Could you check a few things on this model? Use its own coordinates, in mm. A direction names the side the tool comes from. Coordinates: 2 decimals unless noted, no trailing zeros. Loops run counter-clockwise (first coordinate to the right, second up) from the corner with the lowest first, then second, coordinate; pieces in that order, holes last.
1) Imagine slicing it at A-A on x = -15.5. Please give me the cut outline in (y, z).
2) Will these pins go through, and if not, where does the flat tip stop? P1, Ø5, axis at x = -12, y = 40.5, coming from the +Z side; P2, Ø3, axis at x = 15.5, z = -5.5, coming from the +Y side.
3) For faces 4 (the face through (-28, 13, 10)), 5 (the face through (11.15, 53, 12)), 6 (the face through (-31.458, 33.247, -1.689)), 7 (the face through (17.235, 53.028, -5.728)), 8 (the face through (0, 3, 2)), which set-ups out of +Z, -Z, +X, -X, +Y, -Y let a thin tool reach every point of the face, with its end or its side?
4) If I drill on line 1 along X through (y, z) = (53.1, -5.5); line 2 along Y through (x, z) = (13, -9.5); line 3 along X through (y, z) = (17.5, 9.5), over which ranges is the centre line in solid material (lowest first)?
5) Imagine slicing it at C-C on x = 0. Please give me the cut outline in (y, z).
6) Thinking about a two-plate mould opening in Y: for faces 1 (the face through (0, 0, 0)), 2 (the face through (-0.245, 52.986, -1.147)), 3 (the face through (0, 51, -5)), which applies, released by +Y, released by -Y, zero draft, split by the parting line, or undercut?
7) Imagine slicing it at D-D on y = 41. Please give me the cut outline in (x, z).
8) Imagine slicing it at B-B on z = -10. Please give me the cut outline in (x, y).
```python
from build123d import *

# Parameters (mm, degrees)
CROQUIS1_W              = 70
CROQUIS1_H              = 30
SALIENTE_EXTRUIR1_DEPTH = 55
CROQUIS5_W              = 44
CROQUIS5_H              = 48
CORTAR_EXTRUIR3_DEPTH   = 27
CORTAR_EXTRUIR4_REACH   = 65.647
CROQUIS6_R              = 11.15
CORTAR_EXTRUIR5_START   = -4
CROQUIS7_W              = 22.3
CROQUIS7_H              = 5
CORTAR_EXTRUIR5_DEPTH   = 4
CROQUIS9_R              = 4.15
CORTAR_EXTRUIR6_DEPTH   = 27
REDONDEO1_R             = 1
CORTAR_EXTRUIR7_DEPTH   = 1
CORTAR_EXTRUIR8_REACH   = 68.895
CROQUIS11_R             = 1.75
CORTAR_EXTRUIR9_REACH   = 82.616


with BuildPart() as part:
    # Croquis1 → Saliente-Extruir1 (new body)
    with BuildSketch(Plane(origin=(0, 0, 0), x_dir=(1, 0, 0), z_dir=(0, 1, 0))):
        Rectangle(CROQUIS1_W, CROQUIS1_H)
    extrude(amount=SALIENTE_EXTRUIR1_DEPTH)

    # Croquis5 → Cortar-Extruir3 (cut)
    with BuildSketch(Plane.XY.offset(15)):
        with Locations((0, 27)):
            Rectangle(CROQUIS5_W, CROQUIS5_H)
    extrude(amount=-CORTAR_EXTRUIR3_DEPTH, mode=Mode.SUBTRACT)

    # Croquis6 → Cortar-Extruir4 (cut, up to next)
    with BuildSketch(Plane.XZ.offset(-51), mode=Mode.PRIVATE) as cortar_extruir4_sk1:
        with Locations((0, 10)):
            Circle(CROQUIS6_R)
    cortar_extruir4_tool1 = extrude(cortar_extruir4_sk1.sketch, amount=-CORTAR_EXTRUIR4_REACH, mode=Mode.PRIVATE) & part.part
    add(cortar_extruir4_tool1.solids().sort_by_distance((0, 51, 10))[0], mode=Mode.SUBTRACT)

    # Croquis7 → Cortar-Extruir5 (cut)
    with BuildSketch(Plane(origin=(0, 55, 0), x_dir=(1, 0, 0), z_dir=(0, 1, 0)).offset(CORTAR_EXTRUIR5_START)):
        with Locations((0, -12.5)):
            Rectangle(CROQUIS7_W, CROQUIS7_H)
    extrude(amount=CORTAR_EXTRUIR5_DEPTH, mode=Mode.SUBTRACT)

    # Croquis9 → Cortar-Extruir6 (cut)
    with BuildSketch(Plane(origin=(0, 0, -15), x_dir=(-1, 0, 0), z_dir=(0, 0, -1))):
        with Locations((-27.5, 32)):
            Circle(CROQUIS9_R)
        with Locations((27.5, 32)):
            Circle(CROQUIS9_R)
    extrude(amount=-CORTAR_EXTRUIR6_DEPTH, mode=Mode.SUBTRACT)

    # Redondeo1
    redondeo1_edges = [part.edges().sort_by_distance(p)[0] for p in [
        (-35, 55, 0),
        (-23.075, 55, 15),
        (-22, 27, 15),
        (0, 3, 15),
        (22, 27, 15),
        (16.575, 51, 15),
        (0, 55, -1.15),
        (23.075, 55, 15),
        (11.15, 51, 12.5),
        (35, 55, 0),
        (11.15, 55, 12.5),
        (11.15, 53, 15),
        (0, 51, -1.15),
        (-16.575, 51, 15),
        (-11.15, 51, 12.5),
        (-11.15, 55, 12.5),
        (-11.15, 53, 15),
        (0, 55, -15),
        (35, 27.5, 15),
        (-35, 27.5, 15),
        (-35, 27.5, -15),
        (35, 27.5, -15),
    ]]
    fillet(redondeo1_edges, radius=REDONDEO1_R)

    # Croquis10 → Cortar-Extruir7 (cut)
    with BuildSketch(Plane.XY.offset(15)):
        with BuildLine():
            Line((30.192307692, 11.128219757), (30.192307692, 10.512835142))
            Line((30.192307692, 10.512835142), (28.151442308, 10.512835142))
            Line((28.151442308, 10.512835142), (27.828125, 8.934710142))
            add(Edge.make_bspline(
                [(27.828125, 8.934710142), (27.891649356, 8.952247751), (28.014717749, 8.986224094), (28.196363225, 9.023948272), (28.368807002, 9.046689033), (28.480707637, 9.049794137), (28.534855769, 9.05129668)],
                knots=[0, 0, 0, 0, 1.100273476, 2.13160584, 3.095893838, 4, 4, 4, 4], degree=3))
            add(Edge.make_bspline(
                [(28.534855769, 9.05129668), (28.601856466, 9.049846505), (28.733596576, 9.046995098), (28.926349056, 9.019614784), (29.110348302, 8.976517788), (29.285209508, 8.916311179), (29.451256166, 8.839323065), (29.606960557, 8.743151739), (29.754659836, 8.630808885), (29.891704283, 8.501646008), (30.016031669, 8.359494665), (30.125344794, 8.2066526), (30.218194949, 8.044605179), (30.292870528, 7.871804136), (30.352500816, 7.690159873), (30.39218995, 7.49776116), (30.418618594, 7.296421525), (30.421571256, 7.158756548), (30.423076923, 7.088556296)],
                knots=[0, 0, 0, 0, 1.052922333, 2.070308379, 3.05430497, 4.020497103, 4.973039431, 5.925935799, 6.892292201, 7.88610001, 8.88166317, 9.857072816, 10.836096531, 11.812156883, 12.81219415, 13.836441305, 14.89672472, 16, 16, 16, 16], degree=3))
            add(Edge.make_bspline(
                [(30.423076923, 7.088556296), (30.421936794, 7.039661061), (30.419671944, 6.942531368), (30.408154365, 6.798284167), (30.385978852, 6.657090739), (30.35620561, 6.518932353), (30.317561465, 6.384070572), (30.27078023, 6.252119381), (30.213529897, 6.123900055), (30.150733254, 5.998199378), (30.080025006, 5.87785908), (30.001547565, 5.76531796), (29.918635294, 5.658887763), (29.82942149, 5.559709935), (29.733076927, 5.46843619), (29.630768413, 5.384524851), (29.523312323, 5.306556856), (29.409046193, 5.237697093), (29.290516222, 5.174332025), (29.166010707, 5.122348818), (29.038363792, 5.075873627), (28.905738291, 5.038828723), (28.768434612, 5.009801486), (28.626226426, 4.990086171), (28.479859563, 4.975726564), (28.380645256, 4.974827666), (28.330528846, 4.974373604)],
                knots=[0, 0, 0, 0, 1.056347294, 2.098418968, 3.122841568, 4.141288669, 5.149314143, 6.15115421, 7.162517403, 8.180376062, 9.185164535, 10.17417709, 11.141909838, 12.097768115, 13.052685741, 14.0056014, 14.954263652, 15.917497458, 16.885230207, 17.854509472, 18.828990115, 19.81800267, 20.826176721, 21.857883937, 22.917946725, 24, 24, 24, 24], degree=3))
            add(Edge.make_bspline(
                [(28.330528846, 4.974373604), (28.270744536, 4.975557897), (28.153125969, 4.977887855), (27.980804997, 5.002262401), (27.81500853, 5.037171972), (27.657071214, 5.089691292), (27.505577619, 5.155498083), (27.362567246, 5.238668663), (27.224385916, 5.332918555), (27.096650995, 5.444142017), (26.978097658, 5.565711758), (26.871972214, 5.697639142), (26.777457511, 5.837746757), (26.696067088, 5.986715022), (26.626641908, 6.144152503), (26.572101929, 6.310649076), (26.528081891, 6.485334797), (26.509458885, 6.605597958), (26.5, 6.666681296)],
                knots=[0, 0, 0, 0, 1.0467383, 2.05933395, 3.04377827, 4.011590433, 4.970194871, 5.932262533, 6.905835911, 7.896367577, 8.894135286, 9.877477877, 10.858688626, 11.851381753, 12.8477658, 13.868841284, 14.917554742, 16, 16, 16, 16], degree=3))
            Line((26.5, 6.666681296), (27.038461538, 6.666681296))
            add(Edge.make_bspline(
                [(27.038461538, 6.666681296), (27.051710494, 6.60946452), (27.077175722, 6.4994907), (27.133071291, 6.34497983), (27.201412792, 6.207289732), (27.28267739, 6.084599018), (27.379620299, 5.977612165), (27.490242177, 5.88226863), (27.614266845, 5.796254123), (27.75208381, 5.724557951), (27.897477661, 5.663411516), (28.049650021, 5.622694325), (28.204457472, 5.594064223), (28.309163249, 5.591198347), (28.361778846, 5.589758219)],
                knots=[0, 0, 0, 0, 1.136247022, 2.183929868, 3.172523383, 4.106158343, 5.02341133, 5.958108904, 6.928429099, 7.938127109, 8.96079061, 9.975095812, 10.982467395, 12, 12, 12, 12], degree=3))
            add(Edge.make_bspline(
                [(28.361778846, 5.589758219), (28.413136179, 5.591165267), (28.514259189, 5.593935755), (28.663078709, 5.615259776), (28.806757922, 5.648101327), (28.943879105, 5.69724965), (29.076841744, 5.756983453), (29.202282493, 5.833637869), (29.323830283, 5.921855043), (29.437707083, 6.022923552), (29.542003282, 6.134300171), (29.634156632, 6.253404274), (29.710917055, 6.380461725), (29.775604099, 6.513272844), (29.82472404, 6.653293228), (29.859765722, 6.799866671), (29.880342394, 6.953355209), (29.883172989, 7.058045454), (29.884615385, 7.111392834)],
                knots=[0, 0, 0, 0, 1.027316725, 2.022795036, 3.002884548, 3.971462791, 4.93288096, 5.914575861, 6.907176829, 7.935150275, 8.956128384, 9.956726525, 10.942570165, 11.921478529, 12.907843606, 13.90538589, 14.932640048, 16, 16, 16, 16], degree=3))
            add(Edge.make_bspline(
                [(29.884615385, 7.111392834), (29.883486563, 7.159522694), (29.881277054, 7.253730047), (29.863224648, 7.391557258), (29.831824124, 7.521968188), (29.78824033, 7.645592589), (29.732904031, 7.762547061), (29.665281781, 7.872952307), (29.584104528, 7.975353164), (29.491375576, 8.069797542), (29.389790363, 8.156960185), (29.27760109, 8.231264333), (29.157155501, 8.293773906), (29.029904759, 8.347719046), (28.892822076, 8.386463181), (28.748622134, 8.415550985), (28.595747778, 8.432377321), (28.491226598, 8.434711986), (28.4375, 8.435912065)],
                knots=[0, 0, 0, 0, 1.045622112, 2.046656509, 3.013763289, 3.955457236, 4.890082067, 5.820317437, 6.762574623, 7.722996705, 8.69280354, 9.665887285, 10.63943826, 11.638615906, 12.663482002, 13.728887084, 14.832589034, 16, 16, 16, 16], degree=3))
            add(Edge.make_bspline(
                [(28.4375, 8.435912065), (28.390993265, 8.434916766), (28.294968656, 8.432861726), (28.147672381, 8.417730588), (27.992886571, 8.393320369), (27.831204578, 8.359743945), (27.66214085, 8.315804956), (27.486052163, 8.263151527), (27.302568277, 8.200199529), (27.178937893, 8.152658591), (27.115384615, 8.128219757)],
                knots=[0, 0, 0, 0, 0.817624296, 1.688186739, 2.600797293, 3.572016777, 4.590301741, 5.671205678, 6.80286297, 8, 8, 8, 8], degree=3))
            Line((27.115384615, 8.128219757), (27.730769231, 11.128219757))
            Line((27.730769231, 11.128219757), (30.192307692, 11.128219757))
        make_face()
    extrude(amount=-CORTAR_EXTRUIR7_DEPTH, mode=Mode.SUBTRACT)

    # Croquis11 → Cortar-Extruir8 (cut, up to next)
    with BuildSketch(Plane(origin=(0, 55, 0), x_dir=(1, 0, 0), z_dir=(0, 1, 0)), mode=Mode.PRIVATE) as cortar_extruir8_sk1:
        with Locations(Location((-15.5, 5.5, 0), (0, 0, 270))):
            Circle(CROQUIS11_R)
    cortar_extruir8_tool1 = extrude(cortar_extruir8_sk1.sketch, amount=-CORTAR_EXTRUIR8_REACH, mode=Mode.PRIVATE) & part.part
    # Croquis11 → Cortar-Extruir8 (cut, up to next)
    with BuildSketch(Plane(origin=(0, 55, 0), x_dir=(1, 0, 0), z_dir=(0, 1, 0)), mode=Mode.PRIVATE) as cortar_extruir8_sk2:
        with Locations(Location((15.5, 5.5, 0), (0, 0, 270))):
            Circle(CROQUIS11_R)
    cortar_extruir8_tool2 = extrude(cortar_extruir8_sk2.sketch, amount=-CORTAR_EXTRUIR8_REACH, mode=Mode.PRIVATE) & part.part
    add(cortar_extruir8_tool1.solids().sort_by_distance((-15.5, 55, -5.5))[0], mode=Mode.SUBTRACT)
    add(cortar_extruir8_tool2.solids().sort_by_distance((15.5, 55, -5.5))[0], mode=Mode.SUBTRACT)

    # Croquis14 → Cortar-Extruir9 (cut, up to next)
    with BuildSketch(Plane(origin=(-22, 0, 0), x_dir=(0, 0, -1), z_dir=(1, 0, 0)), mode=Mode.PRIVATE) as cortar_extruir9_sk1:
        with BuildLine():
            Line((-15, 3), (-5, 3))
            add(Edge.make_bspline(
                [(-5, 3), (-3.519296534, 3), (-3.519296534, 8), (-3.519296534, 13), (-5, 13)],
                knots=[3.141592654, 3.141592654, 3.141592654, 4.71238898, 4.71238898, 6.283185307, 6.283185307, 6.283185307], degree=2, weights=[1, 0.707106781, 1, 0.707106781, 1]))
            Line((-5, 13), (-15, 13))
            Line((-15, 13), (-15, 3))
        make_face()
    cortar_extruir9_tool1 = extrude(cortar_extruir9_sk1.sketch, amount=-CORTAR_EXTRUIR9_REACH, mode=Mode.PRIVATE) & part.part
    add(cortar_extruir9_tool1.solids().sort_by_distance((-22, 8, 9.413236))[0], mode=Mode.SUBTRACT)


solid = part.part
```
Filled in:
1. outline: (0, -15) - (54, -15) arc R1 ccw to (55, -14) - (55, -7.25) - (51, -7.25) - (51, -12) - (3, -12) - (3, 14) arc R1 ccw to (2, 15) - (0, 15) - close; (51, -3.75) - (55, -3.75) - (55, 14) arc R1 ccw to (54, 15) - (52, 15) arc R1 ccw to (51, 14) - close
2. P1: stops at z = -12
2. P2: stops at y = 3
3. face 4: +Z, -X
3. face 5: +Z, +Y
3. face 6: -Z
3. face 7: +Y
3. face 8: +Z
4. line 1: x = -35 to -17.25, -13.75 to 13.75, 17.25 to 35
4. line 2: y = 0 to 3, 51 to 55
4. line 3: x = -35 to -22, 22 to 35
5. outline: (0, -15) - (54, -15) arc R1 ccw to (55, -14) - (55, -2.15) arc R1 ccw to (54, -1.15) - (52, -1.15) arc R1 ccw to (51, -2.15) - (51, -12) - (3, -12) - (3, 14) arc R1 ccw to (2, 15) - (0, 15) - close
6. face 1: released by -Y
6. face 2: zero draft
6. face 3: undercut
7. outline: (-35, -14) arc R1 ccw to (-34, -15) - (34, -15) arc R1 ccw to (35, -14) - (35, 14) arc R1 ccw to (34, 15) - (23, 15) arc R1 ccw to (22, 14) - (22, -12) - (-22, -12) - (-22, 14) arc R1 ccw to (-23, 15) - (-34, 15) arc R1 ccw to (-35, 14) - close
8. outline: (-35, 0) - (35, 0) - (35, 54) arc R1 ccw to (34, 55) - (-34, 55) arc R1 ccw to (-35, 54) - close; hole circle Ø8.3 at (-27.5, 32); hole (-22, 3) - (22, 3) - (22, 51) - (-22, 51) - close; hole circle Ø8.3 at (27.5, 32)
